Could you check a few things on this model? Use its own coordinates, in mm. Face numbers are marked on the shaded views. A direction names the side the tool comes from. Coordinates: 2 decimals unless noted, no trailing zeros. Order: outer loops, then holes, each group sorted by start corner. A loop starts at its lowest first (then second) coordinate and runs counter-clockwise, first axis right, second up. Notation, with made-up numbers: (64, 72.5) - (86, 72.5) arc R15 cw to (86, 84.5) - close; hole circle Ø1 at (-20, 6.5). An arc over 180 degrees is marked (long way). One line per item, written item: value.
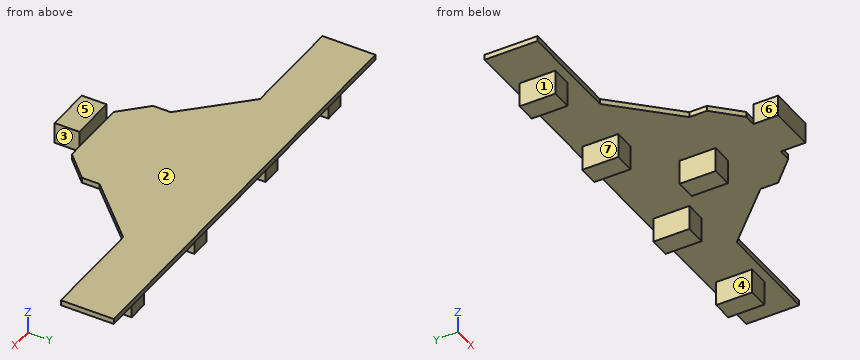
from build123d import *

# Parameters (mm, degrees)
PAD005002_DEPTH = 1.5
SKETCH011_W     = 5.8
SKETCH011_H     = 10.2
PAD005003_DEPTH = 7
SKETCH012_W     = 13
SKETCH012_H     = 7
PAD005004_DEPTH = 6


with BuildPart() as part:
    # Sketch010 → Pad005002 (new body)
    with BuildSketch(Plane.XY):
        Polygon((-62.5, 25), (62.5, 25), (62.5, 10), (32.686661, 10), (17, -6), (17, -11), (10, -18), (-10, -18), (-17, -11), (-17, -6), (-32.686661, 10), (-62.5, 10), align=None)
    extrude(amount=PAD005002_DEPTH)

    # Sketch011 (on Face13 of Pad005002) → Pad005003 (join)
    with BuildSketch(Plane(origin=(0, 0, 0), x_dir=(1, 0, 0), z_dir=(0, 0, -1))):
        Rectangle(SKETCH011_W, SKETCH011_H)
        with Locations((-47, -17.497188)):
            Rectangle(SKETCH011_W, SKETCH011_H)
        with Locations((-17, -17.497188)):
            Rectangle(SKETCH011_W, SKETCH011_H)
        with Locations((17, -17.497188)):
            Rectangle(SKETCH011_W, SKETCH011_H)
        with Locations((47, -17.497188)):
            Rectangle(SKETCH011_W, SKETCH011_H)
    extrude(amount=PAD005003_DEPTH)

    # Sketch012 → Pad005004 (join)
    with BuildSketch(Plane.XY):
        with Locations((-0.091507, -21.5)):
            Rectangle(SKETCH012_W, SKETCH012_H)
    extrude(amount=PAD005004_DEPTH)


with BuildPart() as part_1:
    # Body003002 placement: moved
    add(part.part.moved(Location((0, -93.5, 0))))


solid = part_1.part
Item 1: I want a section at C-C on x = -35. Please give me the cut outline in (y, z).
Conclusion:
outline: (-83.5, 0) - (-68.5, 0) - (-68.5, 1.5) - (-83.5, 1.5) - close
Item 2: Thinking about a two-plate mould opening in X: for the marked faces 5, 6 and 7, which applies, pulls with the +X half, pulls with the -X half, needs draft (parallel to the pull), parting line crosses it, or undercut?
Conclusion:
face 5: needs draft
face 6: pulls with the -X half
face 7: undercut
Item 3: I want a section at B-B on y = -75.5. Please give me the cut outline in (x, z), then the cut area to 3 significant figures.
Conclusion:
outline: (-62.5, 0) - (-49.9, 0) - (-49.9, -7) - (-44.1, -7) - (-44.1, 0) - (-19.9, 0) - (-19.9, -7) - (-14.1, -7) - (-14.1, 0) - (14.1, 0) - (14.1, -7) - (19.9, -7) - (19.9, 0) - (44.1, 0) - (44.1, -7) - (49.9, -7) - (49.9, 0) - (62.5, 0) - (62.5, 1.5) - (-62.5, 1.5) - close
area: 350 mm²
Item 4: For the marked faces 1, 2, 3 and 4, which set-ups out of +Z, -Z, +X, -X, +Y, -Y let a thin tool reach every point of the face, with its end or its side?
Conclusion:
face 1: -Z, -X, +Y, -Y
face 2: +Z, +X, -X, +Y
face 3: +Z, -Z, +X, -Y
face 4: -Z, +Y, -Y
Item 5: If I drill on probe 1 along X at (y, z) = (-79.5, -2.75); probe 2 along X at (y, z) = (-97.5, -1); probe 3 along X at (y, z) = (-116, 1.75), over which ranges is the centre line in solid material (lowest first)?
Conclusion:
probe 1: -49.9 to -44.1, -19.9 to -14.1, 14.1 to 19.9, 44.1 to 49.9
probe 2: -2.9 to 2.9
probe 3: -6.59 to 6.41
Item 6: I'm going to push flat-ended pins straight in: pin 1 Ø13 at (x, y) = (2.5, -93) entering from +Z; pin 2 Ø6 at (x, y) = (1.5, -82) entering from -Z; pin 3 Ø6.5 at (x, z) = (1, -4) entering from -Y. Where does each tip first touch, or does it pass through?
Conclusion:
pin 1: z = 1.5
pin 2: z = 0
pin 3: y = -98.6
Item 7: I want a section at D-D on z = 4. Please give me the cut outline in (x, y).
Conclusion:
outline: (-6.59, -118.5) - (6.41, -118.5) - (6.41, -111.5) - (-6.59, -111.5) - close
Item 8: I want a section at A-A on z = -1.75. Please give me the cut outline in (x, y), then the cut area to 3 significant figures.
Conclusion:
outline: (-49.9, -81.1) - (-44.1, -81.1) - (-44.1, -70.9) - (-49.9, -70.9) - close; (-19.9, -81.1) - (-14.1, -81.1) - (-14.1, -70.9) - (-19.9, -70.9) - close; (-2.9, -98.6) - (2.9, -98.6) - (2.9, -88.4) - (-2.9, -88.4) - close; (14.1, -81.1) - (19.9, -81.1) - (19.9, -70.9) - (14.1, -70.9) - close; (44.1, -81.1) - (49.9, -81.1) - (49.9, -70.9) - (44.1, -70.9) - close
area: 296 mm²
